from build123d import *

# Parameters (mm, degrees)
F1_DEPTH  = 6.35
F2_W      = 25.4
F2_H      = 10.16
F3_DEPTH  = 1.27
F4_R      = 2.54
F5_DEPTH  = 25.4
F6_R      = 2.54
F7_DEPTH  = 25.4
F8_W      = 25.4
F8_H      = 10.16
F8_W_2    = 25.950329153
F9_DEPTH  = 1.27
F10_R     = 2.54
F11_DEPTH = 25.4
F12_R     = 2.54
F13_DEPTH = 25.4
F14_R     = 1.26999


# Not quite as in the source:
# - a fillet or chamfer is up to 0.001 mm smaller than in the source, because OpenCascade refuses the exact size


with BuildPart() as f1:
    # F0 (on Top) → F1 (new body)
    with BuildSketch(Plane.XY):
        Polygon((-53.3815915518, 5.5359576059), (-101.6415915518, 5.5359576059), (-101.6415915518, -51.6140423941), (-53.3815915518, -51.6140423941), (86.3184084482, -51.6140423941), (134.5784084482, -51.6140423941), (134.5784084482, 5.5359576059), (86.3184084482, 5.5359576059), align=None)
    extrude(amount=F1_DEPTH)

    # F2 (on face) → F3 (cut)
    with BuildSketch(Plane.XY.offset(6.35)):
        with Locations((-88.9415915518, 0.4559576059)):
            Rectangle(F2_W, F2_H)
        with Locations((121.8784084482, 0.4559576059)):
            Rectangle(F2_W, F2_H)
    extrude(amount=-F3_DEPTH, mode=Mode.SUBTRACT)

    # F4 (on face) → F5 (cut)
    with BuildSketch(Plane.XY.offset(5.08)):
        with Locations((-97.8315915518, 0.4559576059)):
            Circle(F4_R)
        with Locations((-81.0675915518, 0.4559576059)):
            Circle(F4_R)
    extrude(amount=-F5_DEPTH, mode=Mode.SUBTRACT)

    # F6 (on face) → F7 (cut)
    with BuildSketch(Plane.XY.offset(5.08)):
        with Locations((130.7684084482, 0.4559576059)):
            Circle(F6_R)
        with Locations((114.0044084482, 0.4559576059)):
            Circle(F6_R)
    extrude(amount=-F7_DEPTH, mode=Mode.SUBTRACT)

    # F8 (on face) → F9 (cut)
    with BuildSketch(Plane(origin=(0, 0, 0), x_dir=(1, 0, 0), z_dir=(0, 0, -1))):
        with Locations((-88.9415915518, 46.5340423941)):
            Rectangle(F8_W, F8_H)
        with Locations((121.6032438717, 46.5340423941)):
            Rectangle(F8_W_2, F8_H)
    extrude(amount=-F9_DEPTH, mode=Mode.SUBTRACT)

    # F10 (on face) → F11 (cut)
    with BuildSketch(Plane(origin=(0, 0, 1.27), x_dir=(1, 0, 0), z_dir=(0, 0, -1))):
        with Locations((-97.8315915518, 46.5340423941)):
            Circle(F10_R)
        with Locations((-81.0675915518, 46.5340423941)):
            Circle(F10_R)
    extrude(amount=-F11_DEPTH, mode=Mode.SUBTRACT)

    # F12 (on face) → F13 (cut)
    with BuildSketch(Plane(origin=(0, 0, 1.27), x_dir=(1, 0, 0), z_dir=(0, 0, -1))):
        with Locations((114.0044084482, 46.5340423941)):
            Circle(F12_R)
        with Locations((130.7684084482, 46.5340423941)):
            Circle(F12_R)
    extrude(amount=-F13_DEPTH, mode=Mode.SUBTRACT)

    # F14 (radius 1.27 in the source; OpenCascade refuses exactly that, so slightly less here)
    f14_edges = [f1.edges().sort_by_distance(p)[0] for p in [
        (134.578408, -28.119042, 6.35),
        (134.578408, -17.959042, 0),
        (-101.641592, -28.119042, 6.35),
        (-101.641592, -17.959042, 0),
    ]]
    fillet(f14_edges, radius=F14_R)


solid = f1.part
Input: part model. Units: mm. Frame: model coordinates. A direction names the side the tool comes from. Round coordinates to 2 decimals unless told otherwise and drop trailing zeros. Answer as CSV lines item,"result". Start each with the question number.
(1) Reachability of faces 4 (the flat face through (122, 1, 5.08)), 5 (the flat face through (121, -47, 1.27)), 6 (the flat face through (-89, -47, 1.27)) from +Z, -Z, +X, -X, +Y, -Y: full face, straight path, thin tool, end or side. Return the list, or none.
(2) Draft query along Y for faces 1 (the cylindrical face through (-83.083, -44.988, 3.774)), 2 (the flat face through (18, 5.536, 3)), 3 (the flat face through (134.578, -23, 3)). Return one class per face: released by +Y, released by -Y, zero draft, split by the parting line, or undercut.
(3) Line query: line 1 (X direction, y = -44.5, z = 4.5); line 2 (X direction, y = -48, z = 4.75); line 3 (X direction, y = -42.5, z = 5.25). Output: solid intervals per line, ascending. Write a range as [from, to].
(4) First-contact query: pin 1 (8 mm diameter, centred on x = 124.5, y = -45.5, fed in from -Z); pin 2 (8 mm diameter, centred on x = 122, y = -0.5, fed in from +Z); pin 3 (6 mm diameter, centred on x = 130.77, y = -46.53, fed in from +Z); pin 4 (4.5 mm diameter, centred on x = 114, y = 0.46, fed in from +Z). Flat tips, straight axial feed; report the tip coordinate or a pass-through.
Values found:
1,face 4,"+Z, +X, +Y"
1,face 5,"-Z, +X, -Y"
1,face 6,"-Z, -X, -Y"
2,face 1,"undercut"
2,face 2,"released by +Y"
2,face 3,"zero draft"
3,line 1,"x = [-101.64, -99.35], [-96.31, -82.59], [-79.55, 112.48], [115.53, 129.25], [132.29, 134.58]"
3,line 2,"x = [-101.64, -99.91], [-95.76, -83.14], [-78.99, 111.93], [116.08, 128.69], [132.84, 134.58]"
3,line 3,"x = [-101.63, 134.57]"
4,pin 1,"stops at z = 1.27"
4,pin 2,"stops at z = 5.08"
4,pin 3,"stops at z = 6.35"
4,pin 4,"passes through"
